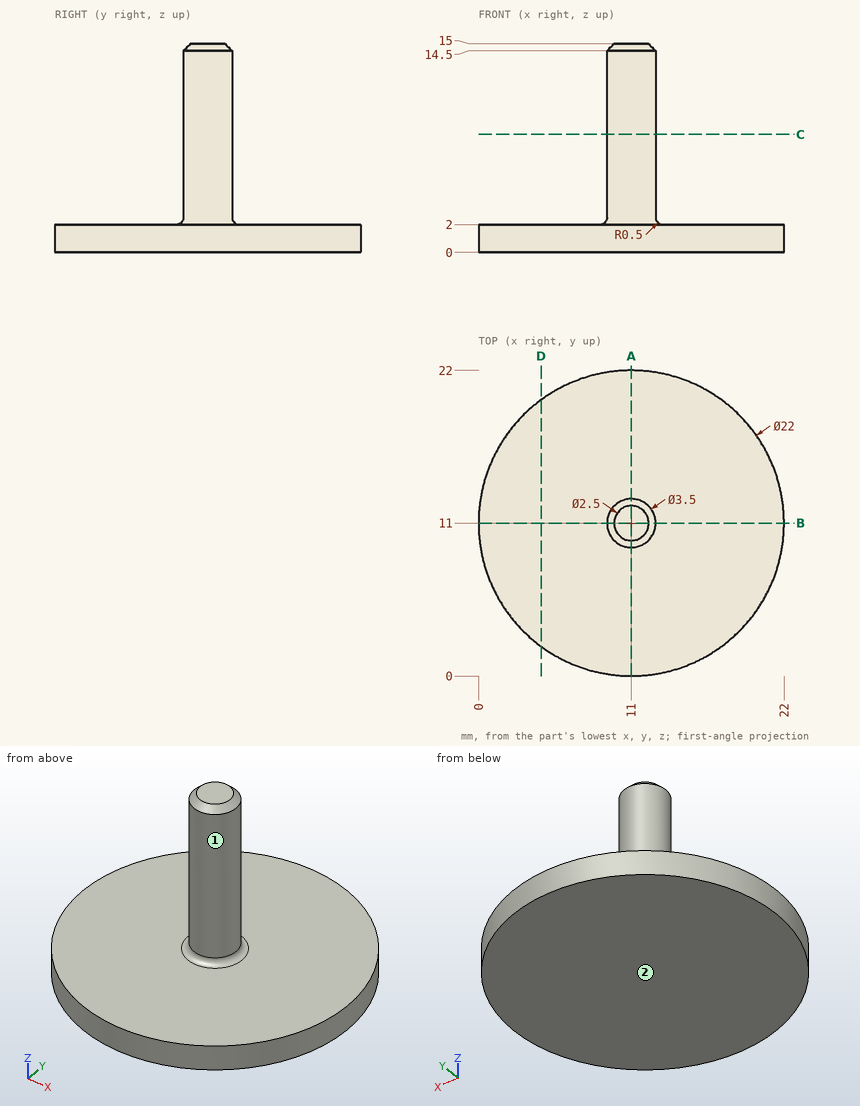
The figure shows three views and two pictorial views of one solid part (mm, origin at its lowest corner). Answer the questions. A direction names the side the tool comes from. Coordinates: 2 decimals unless noted, no trailing zeros. Order: outer loops, then holes, each group sorted by start corner. A loop starts at its lowest first (then second) coordinate and runs counter-clockwise, first axis right, second up.
Q1. Given P1, Ø5, axis at y = 17, z = 7, coming from the +X side; P2, Ø11, axis at x = 7, y = 11, coming from the +Z side; P3, Ø3, axis at y = 12.5, z = 10, coming from the +X side, each flat-ended and moving along its own axis, determine where each tip first touches the part or whether it passes through.
Q2. A cutting plane is placed at A-A, the plane x = 11. Write down the section's boundary in (y, z).
Q3. A cutting plane is placed at C-C, the plane z = 8.5. Write down the section's boundary in (x, y), and give its area (3 significant figures).
Q4. A cutting plane is placed at D-D, the plane x = 4.5. Write down the section's boundary in (y, z), and give its area (3 significant figures).
Q5. Which of the six approach directions +Z, -Z, +X, -X, +Y, -Y give full straight-line access (tool end or side, diameter ignored) to the marked faces 1 and 2?
Q6. Consider line 1 (Z direction, x = 5, y = 17); line 2 (Y direction, x = 11.25, z = 1.25); line 3 (Y direction, x = 11.5, z = 6.75). Determine where each line is inside the solid, lowest interval first.
Answers follow:
1. P1: passes through
1. P2: stops at z = 15
1. P3: stops at x = 12.75
2. outline: (0, 0) - (22, 0) - (22, 2) - (13.25, 2) arc R0.5 cw to (12.75, 2.5) - (12.75, 14.5) - (12.25, 15) - (9.75, 15) - (9.25, 14.5) - (9.25, 2.5) arc R0.5 cw to (8.75, 2) - (0, 2) - close
3. outline: circle Ø3.5 at (11, 11)
3. area: 9.62 mm2
4. outline: (2.13, 0) - (19.87, 0) - (19.87, 2) - (2.13, 2) - close
4. area: 35.5 mm2
5. face 1: +Z
5. face 2: -Z, +X, -X, +Y, -Y
6. line 1: z = 0 to 2
6. line 2: y = 0 to 22
6. line 3: y = 9.32 to 12.68
